Autodesk Inventor part; units mm, degrees
ref_plane "YZ Plane" through (0, 0, 0) normal (1, 0, 0) x (0, 1, 0)
ref_plane "XZ Plane" through (0, 0, 0) normal (0, 1, 0) x (-1, 0, 0)
ref_plane "XY Plane" through (0, 0, 0) normal (0, 0, 1) x (1, 0, 0)
sketch "Sketch1" plane through (0, 0, 0) normal (0, 0, 1) x (1, 0, 0)
  line L0 (-25, 0) -> (25, 0)
  line L1 (25, 0) -> (25, 46.5)
  line L2 (25, 46.5) -> (-25, 46.5)
  line L3 (-25, 46.5) -> (-25, 0)
  circle A0 centre (-12.5, 26.5) radius 3.25
  circle A1 centre (12.5, 26.5) radius 3.25
  point P0 (0, 0)
  dimension "d0" = 50
  dimension "d1" = 46.5
  dimension "d2" = 6.5
  dimension "d3" = 6.5
extrude "Extrusion1" add sketch "Sketch1" along normal blind 6.5
sketch "Sketch2" plane through (0, 0, 6.5) normal (0, 0, 1) x (1, 0, 0)
  line L0 (-25, 0) -> (25, 0)
  line L1 (25, 0) -> (25, 6.5)
  line L2 (25, 6.5) -> (-25, 6.5)
  line L3 (-25, 6.5) -> (-25, 0)
  point P0 (0, 0)
  dimension "d6" = 50
  dimension "d7" = 6.5
extrude "Extrusion2" add sketch "Sketch2" along normal blind 40
sketch "Sketch3" plane through (-25, 6.5, 6.5) normal (0, 1, 0) x (1, 0, 0)
  circle A0 centre (12.5, -26.5) radius 3.25
  circle A1 centre (37.5, -26.5) radius 3.25
  point P0 (25, 6.5)
  dimension "d10" = 6.5
  dimension "d11" = 6.5
hole "Hole1" at (-12.5, 6.5, 33) direction (0, -1, 0) diameter 6.5 end through all
sketch "Sketch4" plane through (-25, 6.5, 6.5) normal (0, 1, 0) x (1, 0, 0)
  circle A0 centre (37.5, -26.5) radius 3.25
  point P0 (25, 6.5)
  dimension "d19" = 6.5
hole "Hole2" at (12.5, 6.5, 33) direction (0, -1, 0) diameter 6.5 end through all
properties part number "Angle"
Verification items for the finished model (mm, model axes). A direction names the side the tool comes from. Coordinates: 2 decimals unless noted, no trailing zeros. Write each loop counter-clockwise with the first axis right and the second up, starting at its lowest first coordinate (ties: lowest second). Pieces come first, ordered by that corner, then holes. Notation, with made-up numbers: (-26, -14) - (-21, -14) arc R33 ccw to (-21, 18) - close; hole circle Ø10 at (48.25, -17.5). An arc over 180 degrees is marked (long way). Answer as a JSON object with one key per item and string values.
(1) Gauge pin test, flat ends, axial feed: pin 1 Ø6 at (x, z) = (12.5, 33) entering from -Y; pin 2 Ø6 at (x, z) = (7, 28) entering from +Y; pin 3 Ø7.5 at (x, y) = (12.5, 26.5) entering from +Z. Record the tip position at first contact, or that the pin passes through.
Report:
{"pin 1": "through", "pin 2": "y = 6.5", "pin 3": "z = 6.5"}
(2) Cross-section at D-D on x = -7.5. Record the cut outline in (y, z).
Report:
{"outline": "(0, 0) - (46.5, 0) - (46.5, 6.5) - (6.5, 6.5) - (6.5, 46.5) - (0, 46.5) - close"}
(3) Cross-section at C-C on y = 25. Record the cut outline in (x, z).
Report:
{"outline": "(-25, 0) - (-15.38, 0) - (-15.38, 6.5) - (-25, 6.5) - close; (-9.62, 0) - (9.62, 0) - (9.62, 6.5) - (-9.62, 6.5) - close; (15.38, 0) - (25, 0) - (25, 6.5) - (15.38, 6.5) - close"}
(4) Tool access check on faces 5 (the flat face through (0, 3, 46.5)), 6 (the flat face through (0, 6.5, 26)). Record the directions out of +Z, -Z, +X, -X, +Y, -Y that give a thin tool (end or side, any length) a straight path to the whole face; none if there is none.
Report:
{"face 5": "+Z, +X, -X, +Y, -Y", "face 6": "+Z, +X, -X, +Y"}
(5) Thickness scan on line 1 along X through (y, z) = (2.25, 33); line 2 along Z through (x, y) = (-12.5, 2.25); line 3 along Y through (x, z) = (18.5, 27). Record the ranges inside material, lowest first.
Report:
{"line 1": "-25 to -15.75, -9.25 to 9.25, 15.75 to 25", "line 2": "0 to 29.75, 36.25 to 46.5", "line 3": "0 to 6.5"}
(6) Cross-section at B-B on x = -12.5. Record the cut outline in (y, z), plus the area to 3 significant figures.
Report:
{"outline": "(0, 0) - (23.25, 0) - (23.25, 6.5) - (6.5, 6.5) - (6.5, 29.75) - (0, 29.75) - close; (0, 36.25) - (6.5, 36.25) - (6.5, 46.5) - (0, 46.5) - close; (29.75, 0) - (46.5, 0) - (46.5, 6.5) - (29.75, 6.5) - close", "area": "478 mm^2"}
(7) Mould release check, pull along X, two halves, no side actions. Record for faces 1 (the flat face through (-25, 13, 6)), 2 (the flat face through (0, 27, 6.5)), 3 (the cylindrical face through (-13.205, 29.673, 3.204)), 4 (the flat face through (25, 13, 6)): pulls with the +X half, pulls with the -X half, needs draft (parallel to the pull), parting line crosses it, or undercut.
Report:
{"face 1": "pulls with the -X half", "face 2": "needs draft", "face 3": "undercut", "face 4": "pulls with the +X half"}
(8) Cross-section at A-A on z = 33. Record the cut outline in (x, y).
Report:
{"outline": "(-25, 0) - (-15.75, 0) - (-15.75, 6.5) - (-25, 6.5) - close; (-9.25, 0) - (9.25, 0) - (9.25, 6.5) - (-9.25, 6.5) - close; (15.75, 0) - (25, 0) - (25, 6.5) - (15.75, 6.5) - close"}
